```python
from build123d import *

# Parameters (mm, degrees)
SKETCH2_W             = 539.75
SKETCH2_H             = 84.069565479
BOSS_EXTRUDE1_DEPTH   = 2.54
EDGE_FLANGE1_DEPTH    = 457.2
CUT_EXTRUDE2_DEPTH    = 279.417450967
F_8_CLEARANCE_HOLE1_D = 4.9149


# Sheet-metal steps are written as plain solids
with BuildPart() as part:
    # Sketch2 → Boss-Extrude1 (new body)
    with BuildSketch(Plane.XY):
        with Locations((0, 21.465217261)):
            Rectangle(SKETCH2_W, SKETCH2_H)
    extrude(amount=BOSS_EXTRUDE1_DEPTH)

    # Edge-Flange1 section (across the edge) → Edge-Flange1 (add)
    with BuildSketch(Plane(origin=(228.6, -22.897046661, 0), x_dir=(0, 0.9961946980917445, -0.08715574274766974), z_dir=(-1, 0, 0))):
        with BuildLine():
            Line((-2.54, 2.327481182), (-2.54, 23.072518818))
            Line((-2.54, 23.072518818), (0, 23.072518818))
            Line((0, 23.072518818), (0, 2.327481182))
            ThreePointArc((0, 2.327481182), (0.667315565, 0.611482055), (2.318624413, -0.202853351))
            Line((2.318624413, -0.202853351), (2.097248827, -2.733187884))
            ThreePointArc((2.097248827, -2.733187884), (-1.205368871, -1.104517073), (-2.54, 2.327481182))
        make_face()
    extrude(amount=EDGE_FLANGE1_DEPTH)

    # Sketch17 → Cut-Extrude2 (cut, through all)
    with BuildSketch(Plane.XY.offset(2.54)):
        with BuildLine():
            Line((-238.125, 63.5), (238.125, 63.5))
            ThreePointArc((238.125, 63.5), (0, 44.45), (-238.125, 63.5))
        make_face()
    extrude(amount=-CUT_EXTRUDE2_DEPTH, mode=Mode.SUBTRACT)

    # #8 Clearance Hole1 (through all)
    with Locations(Plane.XY.offset(2.54)):
        with Locations((-254, 44.45), (-254, 19.05), (-254, -6.35), (254, -6.35), (254, 19.05), (254, 44.45)):
            Hole(F_8_CLEARANCE_HOLE1_D / 2)


solid = part.part
```
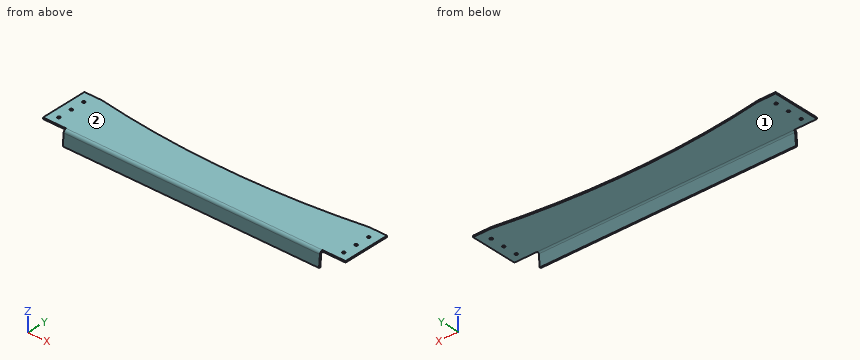
CAD build for the part. Positions are in the model's coordinates, mm. Face numbers are marked on the shaded views. A direction names the side the tool comes from. Coordinates: 2 decimals unless noted, no trailing zeros. Order: outer loops, then holes, each group sorted by start corner. A loop starts at its lowest first (then second) coordinate and runs counter-clockwise, first axis right, second up.
(1) Saw through at D-D, the plane x = -147. Write the cut outline in (y, z).
Solution:
outline: (-27.44, -22.76) - (-24.91, -22.98) - (-23.1, -2.32) arc R2.54 cw to (-20.57, 0) - (51.68, 0) - (51.68, 2.54) - (-20.57, 2.54) arc R5.08 ccw to (-25.63, -2.1) - close
(2) Which spindle directions (+Z, -Z, +X, -X, +Y, -Y) get a long thin tool onto all of the face, cutting with end or side? Do the marked faces 1 and 2. Say none if no direction does.
Solution:
face 1: -Z, +X, -X, +Y
face 2: +Z, +X, -X, +Y, -Y
(3) Saw through at C-C, the plane z = -13.75. Write the cut outline in (x, y), and give its area (3 significant figures).
Solution:
outline: (-228.6, -26.65) - (228.6, -26.65) - (228.6, -24.1) - (-228.6, -24.1) - close
area: 1,170 mm2
(4) Saw through at A-A, the plane x = 148.5. Write the cut outline in (y, z).
Solution:
outline: (-27.44, -22.76) - (-24.91, -22.98) - (-23.1, -2.32) arc R2.54 cw to (-20.57, 0) - (51.83, 0) - (51.83, 2.54) - (-20.57, 2.54) arc R5.08 ccw to (-25.63, -2.1) - close
(5) Pin check, flat tips, straight feed: pin 1 Ø25 at (x, y) = (-6.5, 30.5) entering from -Z; pin 2 Ø7.5 at (y, z) = (-24.5, -6.5) entering from +X; pin 3 Ø12 at (x, z) = (-166.5, -20.5) entering from +Y. Stop position of each tip, or through.
Solution:
pin 1: stops at z = 0
pin 2: stops at x = 228.6
pin 3: stops at y = -24.17
(6) Drill centre lines: L1, parallel to Y at x = 254, z = 0.5; L2, parallel to Z at x = 129, y = 12.5; L3, parallel to Y at x = 172, z = -20.25. Where is each one in solid material? Low to high.
Solution:
L1: y = -20.57 to -8.81, -3.89 to 16.59, 21.51 to 41.99, 46.91 to 63.5
L2: z = 0 to 2.54
L3: y = -27.22 to -24.67
(7) Saw through at B-B, the plane y = 5.5. Write the cut outline in (x, z) (3 decimals), and give its area (3 significant figures).
Solution:
outline: (-269.875, 0) - (269.875, 0) - (269.875, 2.54) - (-269.875, 2.54) - close
area: 1,370 mm2
